```python
from build123d import *

# Parameters (mm, degrees)
F0_W      = 254
F0_H      = 203.2
F1_DEPTH  = 3.175
F2_W      = 51.308
F2_H      = 51.308
F3_DEPTH  = 3.175
F4_W      = 25.908
F4_H      = 25.908
F5_DEPTH  = 3.175
F6_R      = 12.954
F7_DEPTH  = 3.175
F9_DEPTH  = 3.176
F10_R     = 25.654
F11_DEPTH = 3.175
F13_DEPTH = 3.175
F14_R     = 5.08
F15_R     = 5.08
F16_R     = 5.08
F17_R     = 5.08


with BuildPart() as f1:
    # F0 (on Top) → F1 (new body)
    with BuildSketch(Plane.XY):
        with Locations((3.054343, 10.392927)):
            Rectangle(F0_W, F0_H)
    extrude(amount=F1_DEPTH)

    # F2 (on face) → F3 (cut, through all)
    with BuildSketch(Plane.XY.offset(3.175)):
        with Locations((-78.505307, 62.120071)):
            Rectangle(F2_W, F2_H)
    extrude(amount=-F3_DEPTH, mode=Mode.SUBTRACT)

    # F4 (on face) → F5 (cut, through all)
    with BuildSketch(Plane.XY.offset(3.175)):
        with Locations((84.492568, -67.214648)):
            Rectangle(F4_W, F4_H)
    extrude(amount=-F5_DEPTH, mode=Mode.SUBTRACT)

    # F6 (on face) → F7 (cut, through all)
    with BuildSketch(Plane.XY.offset(3.175)):
        with Locations((-71.979322, -61.128017)):
            Circle(F6_R)
    extrude(amount=-F7_DEPTH, mode=Mode.SUBTRACT)

    # F8 (on face) → F9 (cut, through all)
    with BuildSketch(Plane.XY.offset(3.175)):
        Polygon((76.70291, 83.061458), (51.04891, 31.753458), (102.35691, 31.753458), align=None)
    extrude(amount=-F9_DEPTH, mode=Mode.SUBTRACT)

    # F10 (on face) → F11 (cut, through all)
    with BuildSketch(Plane.XY.offset(3.175)):
        with Locations((31.222314, -20.150894)):
            Circle(F10_R)
    extrude(amount=-F11_DEPTH, mode=Mode.SUBTRACT)

    # F12 (on face) → F13 (cut, through all)
    with BuildSketch(Plane.XY.offset(3.175)):
        Polygon((-34.845916, 0), (-47.799916, -25.908), (-21.891916, -25.908), align=None)
    extrude(amount=-F13_DEPTH, mode=Mode.SUBTRACT)

    # F14
    f14_edges = [f1.edges().sort_by_distance(p)[0] for p in [
        (-123.945657, 111.992927, 1.5875),
    ]]
    fillet(f14_edges, radius=F14_R)

    # F15
    f15_edges = [f1.edges().sort_by_distance(p)[0] for p in [
        (130.054343, 111.992927, 1.5875),
    ]]
    fillet(f15_edges, radius=F15_R)

    # F16
    f16_edges = [f1.edges().sort_by_distance(p)[0] for p in [
        (130.054343, -91.207073, 1.5875),
    ]]
    fillet(f16_edges, radius=F16_R)

    # F17
    f17_edges = [f1.edges().sort_by_distance(p)[0] for p in [
        (-123.945657, -91.207073, 1.5875),
    ]]
    fillet(f17_edges, radius=F17_R)


solid = f1.part
```
Check sheet for the modelled part. Datum: model origin and axes. Units: mm. A direction names the side the tool comes from. Give positions to 0.01 mm unless a question says otherwise; leave off trailing zeros. Write each loop counter-clockwise with the first axis right and the second up, starting at its lowest first coordinate (ties: lowest second). Pieces come first, ordered by that corner, then holes. Notation, with made-up numbers: (2, 62.5) - (52, 62.5) arc R32 cw to (52, 94.5) - close; hole circle Ø11 at (-4.75, 83.5). An arc over 180 degrees is marked (long way). Answer as a JSON object with one key per item and string values. Group by question number.
1) Sectioned sample at D-D (y = 60). Record the cut outline in (x, z) (3 decimals).
2) Release check for a two-part mould opening along Y. For faces 3 (the face through (128.606, -89.679, 1.61)), 4 (the face through (1, 12, 0)), 5 (the face through (128.53, 110.54, 1.61)), 6 (the face through (-73.666, -48.284, 1.61)) record: pulls with the +Y half, pulls with the -Y half, needs draft (parallel to the pull), parting line crosses it, or undercut.
3) Sectioned sample at B-B (x = -28.5). Record the cut outline in (y, z) (3 decimals).
4) Thickness scan on probe 1 along X at (y, z) = (-16, 2); probe 2 along X at (y, z) = (-13, 0.8); probe 3 along Y at (x, z) = (74.5, 1.75). Record the ranges inside material, lowest first. Write a range as from..to.
5) Sectioned sample at C-C (z = 1.9). Record the cut outline in (x, y), then the cut area to 3 significant figures.
6) Depth check by flat-ended pin: P1, Ø20.5, axis at x = -71.98, y = -61.13, coming from the -Z side. Enter the tip coordinate at first touch or a pass-through.
7) Access from +Z, -Z, +X, -X, +Y, -Y to the whole of each face (thin tool, end or side, straight path). Record for faces 1 (the face through (-122.497, 110.465, 1.61)), 2 (the face through (-41.23, -12.77, 1.61)).
8) Sectioned sample at A-A (y = -64). Record the cut outline in (x, z) (3 decimals), then the cut area to 3 significant figures.
Geometry results:
{
 "1": {"outline": "(-123.946, 0) - (-104.159, 0) - (-104.159, 3.175) - (-123.946, 3.175) - close; (-52.851, 0) - (65.172, 0) - (65.172, 3.175) - (-52.851, 3.175) - close; (88.234, 0) - (130.054, 0) - (130.054, 3.175) - (88.234, 3.175) - close"},
 "2": {"face 3": "pulls with the -Y half", "face 4": "needs draft", "face 5": "pulls with the +Y half", "face 6": "undercut"},
 "3": {"outline": "(-91.207, 0) - (-25.908, 0) - (-25.908, 3.175) - (-91.207, 3.175) - close; (-12.692, 0) - (111.993, 0) - (111.993, 3.175) - (-12.692, 3.175) - close"},
 "4": {"probe 1": "x = -123.95..-42.85, -26.85..5.91, 56.54..130.05", "probe 2": "x = -123.95..-41.35, -28.35..6.59, 55.86..130.05", "probe 3": "y = -91.21..-80.17, -54.26..31.75, 78.66..111.99"},
 "5": {"outline": "(-123.95, -86.13) arc R5.08 ccw to (-118.87, -91.21) - (124.97, -91.21) arc R5.08 ccw to (130.05, -86.13) - (130.05, 106.91) arc R5.08 ccw to (124.97, 111.99) - (-118.87, 111.99) arc R5.08 ccw to (-123.95, 106.91) - close; hole (-104.16, 36.47) - (-52.85, 36.47) - (-52.85, 87.77) - (-104.16, 87.77) - close; hole circle Ø25.91 at (-71.98, -61.13); hole (-47.8, -25.91) - (-21.89, -25.91) - (-34.85, 0) - close; hole circle Ø51.31 at (31.22, -20.15); hole (51.05, 31.75) - (102.36, 31.75) - (76.7, 83.06) - close; hole (71.54, -80.17) - (97.45, -80.17) - (97.45, -54.26) - (71.54, -54.26) - close", "area": "44,000 mm^2"},
 "6": {"P1": "passes through"},
 "7": {"face 1": "+Z, -Z, -X, +Y", "face 2": "+Z, -Z"},
 "8": {"outline": "(-123.946, 0) - (-84.611, 0) - (-84.611, 3.175) - (-123.946, 3.175) - close; (-59.348, 0) - (71.539, 0) - (71.539, 3.175) - (-59.348, 3.175) - close; (97.447, 0) - (130.054, 0) - (130.054, 3.175) - (97.447, 3.175) - close", "area": "644 mm^2"}
}
